Part model, mm, in its own coordinate system. A direction names the side the tool comes from. Give positions to 0.01 mm unless a question says otherwise; leave off trailing zeros. Order: outer loops, then holes, each group sorted by start corner. A loop starts at its lowest first (then second) coordinate and runs counter-clockwise, first axis right, second up. Notation, with made-up numbers: M 13,-26.75 L 67,-26.75 A21 ccw 67,1.25 Z; hole C 57.25,70 d7. An arc over 180 degrees is marked long. Answer as a JSON object with one key per item and string values.
from build123d import *

# Parameters (mm, degrees)
F0_W     = 40
F0_H     = 75
F1_DEPTH = 133
F2_R     = 10
F3_DEPTH = 19
F4_R     = 10
F6_DEPTH = 53
F5_R     = 3.2
F7_DEPTH = 12.5


with BuildPart() as f1:
    # F0 (on Right) → F1 (new body)
    with BuildSketch(Plane.YZ):
        Rectangle(F0_W, F0_H)
    extrude(amount=F1_DEPTH)

    # F2 (on face) → F3 (join)
    with BuildSketch(Plane(origin=(0, 0, 0), x_dir=(0, -1, 0), z_dir=(-1, 0, 0))):
        with Locations((0, -17.5)):
            Circle(F2_R)
    extrude(amount=F3_DEPTH)

    # F4 (on face) → F6 (join)
    with BuildSketch(Plane.YZ.offset(133)):
        with Locations((0, -17.5)):
            Circle(F4_R)
    extrude(amount=F6_DEPTH)

    # F5 (on Front) → F7 (cut, symmetric)
    with BuildSketch(Plane.XZ):
        with Locations((-11, -17.5)):
            Circle(F5_R)
        with Locations((181, -17.5)):
            Circle(F5_R)
    extrude(amount=F7_DEPTH, both=True, mode=Mode.SUBTRACT)


solid = f1.part
1. Cut at D-D on z = 5.5. Give the cut face in (x, y).
Worked answers:
{"outline": "M 0,-20 L 133,-20 L 133,20 L 0,20 Z"}
2. Cut at A-A on z = -17.5. Give the cut face in (x, y).
Worked answers:
{"outline": "M -19,-10 L -14.2,-10 L -14.2,10 L -19,10 Z; M -7.8,-10 L 0,-10 L 0,-20 L 133,-20 L 133,-10 L 177.8,-10 L 177.8,10 L 133,10 L 133,20 L 0,20 L 0,10 L -7.8,10 Z; M 184.2,-10 L 186,-10 L 186,10 L 184.2,10 Z"}
3. Probe line 1 along X through (y, z) = (-7, -17.5); line 2 along X through (y, z) = (4, -19.5); line 3 along X through (y, z) = (-7.5, -6). List the from-to ranges inside material, lowest first.
Worked answers:
{"line 1": "x = -19 to -14.2, -7.8 to 177.8, 184.2 to 186", "line 2": "x = -19 to -13.5, -8.5 to 178.5, 183.5 to 186", "line 3": "x = 0 to 133"}
4. Cut at C-C on x = -11. Give the cut face in (y, z).
Worked answers:
{"outline": "M -9.47,-20.7 A10 ccw 9.47,-20.7 Z; M -9.47,-14.3 L 9.47,-14.3 A10 ccw Z"}
5. Which spindle directions (+Z, -Z, +X, -X, +Y, -Y) get a long thin tool onto all of the face, cutting with end or side? Do faces 1 (the cylindrical face through (-9.367, -9.237, -21.33)), 2 (the cylindrical face through (159.13, 9.54, -14.5)), 3 (the flat face through (66, 20, -1)). Say none if no direction does.
Worked answers:
{"face 1": "-X", "face 2": "+X", "face 3": "+Z, -Z, +X, -X, +Y"}
6. Pin check, flat tips, straight feed: P1, Ø8, axis at x = 144.5, y = 12, coming from the +Z side; P2, Ø3, axis at y = -1.5, z = 20.5, coming from the -X side; P3, Ø1, axis at y = -8.5, z = 22.5, coming from the +X side. Stop position of each tip, or through.
Worked answers:
{"P1": "stops at z = -11.5", "P2": "stops at x = 0", "P3": "stops at x = 133"}
7. Cut at B-B on y = -3. Give the cut face in (x, z).
Worked answers:
{"outline": "M -19,-27.04 L 0,-27.04 L 0,-37.5 L 133,-37.5 L 133,-27.04 L 186,-27.04 L 186,-7.96 L 133,-7.96 L 133,37.5 L 0,37.5 L 0,-7.96 L -19,-7.96 Z; hole C -11,-17.5 d6.4; hole C 181,-17.5 d6.4"}
8. Two-plate mould, pull along Z, no slides. Class faces 4 (the flat face through (66, 0, -37.5)), 5 (the cylindrical face through (177.8, -0.1, -17.4)), 6 (the flat face through (186, 0, -17)): +Z half, -Z half, draft (parallel to the pull), parting line (faces both ways), or undercut.
Worked answers:
{"face 4": "-Z half", "face 5": "undercut", "face 6": "draft"}
